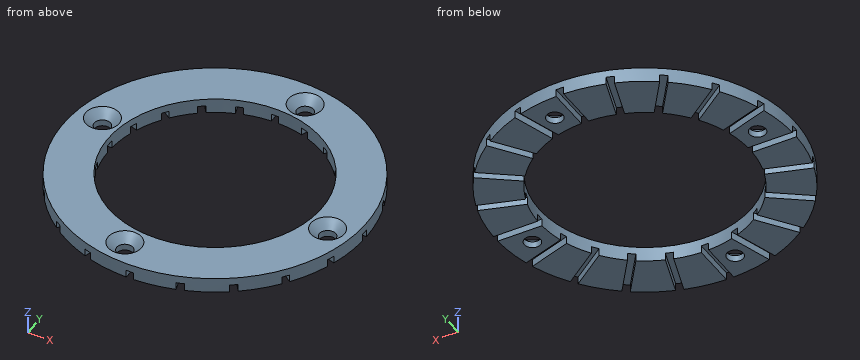
from build123d import *

# Parameters (mm, degrees)
F0_R           = 101.374
F0_R_2         = 71.394
F1_DEPTH       = 10
F3_DEPTH       = 5
F5_D           = 11
F5_CSINK_D     = 22.4
F5_CSINK_ANGLE = 90


with BuildPart() as f1:
    # F0 (on Top) → F1 (new body)
    with BuildSketch(Plane.XY):
        Circle(F0_R)
        Circle(F0_R_2, mode=Mode.SUBTRACT)
    extrude(amount=F1_DEPTH)

    # F2 (on face) → F3 (cut)
    with BuildSketch(Plane(origin=(0, 0, 0), x_dir=(1, 0, 0), z_dir=(0, 0, -1))):
        with BuildLine():
            ThreePointArc((2.5, 101.343168867), (1.2500950523, 101.3662919237), (0, 101.374))
            ThreePointArc((0, 101.374), (-1.2500950523, 101.3662919237), (-2.5, 101.343168867))
            Line((-2.5, 101.343168867), (-2.5, 71.3502153886))
            ThreePointArc((-2.5, 71.3502153886), (0, 71.394), (2.5, 71.3502153886))
            Line((2.5, 71.3502153886), (2.5, 101.343168867))
        make_face()
        with BuildLine():
            ThreePointArc((31.3262879268, 96.4124035626), (30.1349953836, 96.791373217), (28.939120153, 97.1556236189))
            Line((28.939120153, 97.1556236189), (19.6707878167, 68.6306297703))
            ThreePointArc((19.6707878167, 68.6306297703), (22.0619592964, 67.8997289244), (24.4260703981, 67.0855447985))
            Line((24.4260703981, 67.0855447985), (33.6944027344, 95.610538647))
            ThreePointArc((33.6944027344, 95.610538647), (32.5128174779, 96.0187719961), (31.3262879268, 96.4124035626))
        make_face()
        with BuildLine():
            Line((57.5454775947, 83.4578090079), (39.9160618674, 59.1929999324))
            ThreePointArc((39.9160618674, 59.1929999324), (41.9643403022, 57.7589592964), (43.9611468392, 56.254073671))
            Line((43.9611468392, 56.254073671), (61.5905625665, 80.5188827465))
            ThreePointArc((61.5905625665, 80.5188827465), (60.592959405, 81.2722655433), (59.5861417437, 82.0132890945))
            ThreePointArc((59.5861417437, 82.0132890945), (58.5702631175, 82.7418404095), (57.5454775947, 83.4578090079))
        make_face()
        with BuildLine():
            Line((80.5188827465, 61.5905625665), (56.254073671, 43.9611468392))
            ThreePointArc((56.254073671, 43.9611468392), (57.7589592964, 41.9643403022), (59.1929999324, 39.9160618674))
            Line((59.1929999324, 39.9160618674), (83.4578090079, 57.5454775947))
            ThreePointArc((83.4578090079, 57.5454775947), (82.7418395043, 58.5702643962), (82.0132872528, 59.5861442786))
            ThreePointArc((82.0132872528, 59.5861442786), (81.2722646069, 60.592960661), (80.5188827465, 61.5905625665))
        make_face()
        with BuildLine():
            Line((95.610538647, 33.6944027344), (67.0855447985, 24.4260703981))
            ThreePointArc((67.0855447985, 24.4260703981), (67.8997289244, 22.0619592964), (68.6306297703, 19.6707878167))
            Line((68.6306297703, 19.6707878167), (97.1556236189, 28.939120153))
            ThreePointArc((97.1556236189, 28.939120153), (96.7913734751, 30.1349945547), (96.4124040992, 31.3262862756))
            ThreePointArc((96.4124040992, 31.3262862756), (96.0187722746, 32.5128166557), (95.610538647, 33.6944027344))
        make_face()
        with BuildLine():
            Line((101.343168867, 2.5), (71.3502153886, 2.5))
            ThreePointArc((71.3502153886, 2.5), (71.3830530079, 1.2501916945), (71.394, 0))
            ThreePointArc((71.394, 0), (71.3830530079, -1.2501916945), (71.3502153886, -2.5))
            Line((71.3502153886, -2.5), (101.343168867, -2.5))
            ThreePointArc((101.343168867, -2.5), (101.3662919237, -1.2500950523), (101.374, 0))
            ThreePointArc((101.374, 0), (101.3662919237, 1.2500950523), (101.343168867, 2.5))
        make_face()
        with BuildLine():
            Line((97.1556236189, -28.939120153), (68.6306297703, -19.6707878167))
            ThreePointArc((68.6306297703, -19.6707878167), (67.8997289244, -22.0619592964), (67.0855447985, -24.4260703981))
            Line((67.0855447985, -24.4260703981), (95.610538647, -33.6944027344))
            ThreePointArc((95.610538647, -33.6944027344), (96.0187719961, -32.5128174779), (96.4124035626, -31.3262879268))
            ThreePointArc((96.4124035626, -31.3262879268), (96.791373217, -30.1349953836), (97.1556236189, -28.939120153))
        make_face()
        with BuildLine():
            Line((83.4578090079, -57.5454775947), (59.1929999324, -39.9160618674))
            ThreePointArc((59.1929999324, -39.9160618674), (57.7589592964, -41.9643403022), (56.254073671, -43.9611468392))
            Line((56.254073671, -43.9611468392), (80.5188827465, -61.5905625665))
            ThreePointArc((80.5188827465, -61.5905625665), (81.2722651856, -60.5929598848), (82.013288391, -59.586142712))
            ThreePointArc((82.013288391, -59.586142712), (82.7418400637, -58.5702636059), (83.4578090079, -57.5454775947))
        make_face()
        with BuildLine():
            Line((61.5905625665, -80.5188827465), (43.9611468392, -56.254073671))
            ThreePointArc((43.9611468392, -56.254073671), (41.9643403022, -57.7589592964), (39.9160618674, -59.1929999324))
            Line((39.9160618674, -59.1929999324), (57.5454775947, -83.4578090079))
            ThreePointArc((57.5454775947, -83.4578090079), (58.5702643962, -82.7418395043), (59.5861442786, -82.0132872528))
            ThreePointArc((59.5861442786, -82.0132872528), (60.592960661, -81.2722646069), (61.5905625665, -80.5188827465))
        make_face()
        with BuildLine():
            Line((33.6944027344, -95.610538647), (24.4260703981, -67.0855447985))
            ThreePointArc((24.4260703981, -67.0855447985), (22.0619592964, -67.8997289244), (19.6707878167, -68.6306297703))
            Line((19.6707878167, -68.6306297703), (28.939120153, -97.1556236189))
            ThreePointArc((28.939120153, -97.1556236189), (30.1349953836, -96.791373217), (31.3262879268, -96.4124035626))
            ThreePointArc((31.3262879268, -96.4124035626), (32.5128174779, -96.0187719961), (33.6944027344, -95.610538647))
        make_face()
        with BuildLine():
            ThreePointArc((2.5, -71.3502153886), (0, -71.394), (-2.5, -71.3502153886))
            Line((-2.5, -71.3502153886), (-2.5, -101.343168867))
            ThreePointArc((-2.5, -101.343168867), (-1.2500950523, -101.3662919237), (0, -101.374))
            ThreePointArc((0, -101.374), (1.2500950523, -101.3662919237), (2.5, -101.343168867))
            Line((2.5, -101.343168867), (2.5, -71.3502153886))
        make_face()
        with BuildLine():
            ThreePointArc((-19.6707878167, -68.6306297703), (-22.0619592964, -67.8997289244), (-24.4260703981, -67.0855447985))
            Line((-24.4260703981, -67.0855447985), (-33.6944027344, -95.610538647))
            ThreePointArc((-33.6944027344, -95.610538647), (-32.5128191824, -96.018771419), (-31.3262913498, -96.4124024505))
            ThreePointArc((-31.3262913498, -96.4124024505), (-30.1349971018, -96.791372682), (-28.939120153, -97.1556236189))
            Line((-28.939120153, -97.1556236189), (-19.6707878167, -68.6306297703))
        make_face()
        with BuildLine():
            ThreePointArc((-39.9160618674, -59.1929999324), (-41.9643403022, -57.7589592964), (-43.9611468392, -56.254073671))
            Line((-43.9611468392, -56.254073671), (-61.5905625665, -80.5188827465))
            ThreePointArc((-61.5905625665, -80.5188827465), (-60.5929601813, -81.2722649646), (-59.5861433104, -82.0132879563))
            ThreePointArc((-59.5861433104, -82.0132879563), (-58.5702639078, -82.7418398501), (-57.5454775947, -83.4578090079))
            Line((-57.5454775947, -83.4578090079), (-39.9160618674, -59.1929999324))
        make_face()
        with BuildLine():
            ThreePointArc((-56.254073671, -43.9611468392), (-57.7589592964, -41.9643403022), (-59.1929999324, -39.9160618674))
            Line((-59.1929999324, -39.9160618674), (-83.4578090079, -57.5454775947))
            ThreePointArc((-83.4578090079, -57.5454775947), (-82.7418404095, -58.5702631175), (-82.0132890945, -59.5861417437))
            ThreePointArc((-82.0132890945, -59.5861417437), (-81.2722655433, -60.592959405), (-80.5188827465, -61.5905625665))
            Line((-80.5188827465, -61.5905625665), (-56.254073671, -43.9611468392))
        make_face()
        with BuildLine():
            ThreePointArc((-67.0855447985, -24.4260703981), (-67.8997289244, -22.0619592964), (-68.6306297703, -19.6707878167))
            Line((-68.6306297703, -19.6707878167), (-97.1556236189, -28.939120153))
            ThreePointArc((-97.1556236189, -28.939120153), (-96.791373217, -30.1349953836), (-96.4124035626, -31.3262879268))
            ThreePointArc((-96.4124035626, -31.3262879268), (-96.0187719961, -32.5128174779), (-95.610538647, -33.6944027344))
            Line((-95.610538647, -33.6944027344), (-67.0855447985, -24.4260703981))
        make_face()
        with BuildLine():
            ThreePointArc((-71.3502153886, -2.5), (-71.394, 0), (-71.3502153886, 2.5))
            Line((-71.3502153886, 2.5), (-101.343168867, 2.5))
            ThreePointArc((-101.343168867, 2.5), (-101.3662919237, 1.2500950523), (-101.374, 0))
            ThreePointArc((-101.374, 0), (-101.3662919237, -1.2500950523), (-101.343168867, -2.5))
            Line((-101.343168867, -2.5), (-71.3502153886, -2.5))
        make_face()
        with BuildLine():
            ThreePointArc((-68.6306297703, 19.6707878167), (-67.8997289244, 22.0619592964), (-67.0855447985, 24.4260703981))
            Line((-67.0855447985, 24.4260703981), (-95.610538647, 33.6944027344))
            ThreePointArc((-95.610538647, 33.6944027344), (-96.0187717709, 32.5128181431), (-96.4124031286, 31.3262892627))
            ThreePointArc((-96.4124031286, 31.3262892627), (-96.7913730082, 30.1349960542), (-97.1556236189, 28.939120153))
            Line((-97.1556236189, 28.939120153), (-68.6306297703, 19.6707878167))
        make_face()
        with BuildLine():
            ThreePointArc((-59.1929999324, 39.9160618674), (-57.7589592964, 41.9643403022), (-56.254073671, 43.9611468392))
            Line((-56.254073671, 43.9611468392), (-80.5188827465, 61.5905625665))
            ThreePointArc((-80.5188827465, 61.5905625665), (-81.272264828, 60.5929603645), (-82.0132876875, 59.5861436802))
            ThreePointArc((-82.0132876875, 59.5861436802), (-82.741839718, 58.5702640943), (-83.4578090079, 57.5454775947))
            Line((-83.4578090079, 57.5454775947), (-59.1929999324, 39.9160618674))
        make_face()
        with BuildLine():
            ThreePointArc((-43.9611468392, 56.254073671), (-41.9643403022, 57.7589592964), (-39.9160618674, 59.1929999324))
            Line((-39.9160618674, 59.1929999324), (-57.5454775947, 83.4578090079))
            ThreePointArc((-57.5454775947, 83.4578090079), (-58.5702643962, 82.7418395043), (-59.5861442786, 82.0132872528))
            ThreePointArc((-59.5861442786, 82.0132872528), (-60.592960661, 81.2722646069), (-61.5905625665, 80.5188827465))
            Line((-61.5905625665, 80.5188827465), (-43.9611468392, 56.254073671))
        make_face()
        with BuildLine():
            Line((-19.6707878167, 68.6306297703), (-28.939120153, 97.1556236189))
            ThreePointArc((-28.939120153, 97.1556236189), (-30.134995798, 96.791373088), (-31.3262887525, 96.4124032944))
            ThreePointArc((-31.3262887525, 96.4124032944), (-32.5128178891, 96.0187718569), (-33.6944027344, 95.610538647))
            Line((-33.6944027344, 95.610538647), (-24.4260703981, 67.0855447985))
            ThreePointArc((-24.4260703981, 67.0855447985), (-22.0619592964, 67.8997289244), (-19.6707878167, 68.6306297703))
        make_face()
    extrude(amount=-F3_DEPTH, mode=Mode.SUBTRACT)

    # F5 (through all)
    with Locations(Plane.XY.offset(10)):
        with Locations((13.2969295284, 83.9535089506), (83.9535089506, -13.2969295284), (-83.9535089506, 13.2969295284), (-13.2969295284, -83.9535089506)):
            CounterSinkHole(F5_D / 2, F5_CSINK_D / 2, counter_sink_angle=F5_CSINK_ANGLE)


solid = f1.part
Here's how the part is built. I have some questions about the finished solid (model axes, mm). Round coordinates to 2 decimals unless told otherwise and drop trailing zeros. Loops run counter-clockwise (first coordinate to the right, second up) from the corner with the lowest first, then second, coordinate; pieces in that order, holes last. Notation, with made-up numbers: (-38, 35.25) - (8, 35.25) arc R17 cw to (8, 64.25) - close; hole circle Ø9 at (47, 69.25). An arc over 180 degrees is marked (long way). One line per question, with ' | ' between items. Start each with the question number.
Q1. Please list where these lines run through material, in increasing order: line 1 (Y direction, x = 83.5, z = 4.75); line 2 (X direction, y = -82.5, z = 3.5); line 3 (X direction, y = 87, z = 1). Write a range as [from, to].
Q2. I want a section at A-A (y = -52). Write out the boundary of the cut face in (x, z), then the cut area to 3 significant figures.
Q3. I want a section at B-B (z = 7.25). Write out the boundary of the cut face in (x, y), then the cut area to 3 significant figures.
Q4. I want a section at C-C (x = 64.5). Write out the boundary of the cut face in (y, z), then the cut area to 3 significant figures.
Q5. Will these pins go through, and if not, where does the flat tip stop? pin 1 (2.5 mm diameter, centred on y = 91, z = 3.5, fed in from -X); pin 2 (4 mm diameter, centred on x = -65.5, z = 8.5, fed in from +Y); pin 3 (2 mm diameter, centred on y = -61.5, z = 1.5, fed in from -X).
Response values:
1) line 1: y = [-57.48, -29.76], [-24.5, -19.23], [-7.36, -2.5], [2.5, 24.5], [29.76, 57.48] | line 2: x = [-56.85, -29.43], [-24.18, -18.6], [-7.99, -2.5], [2.5, 24.18], [29.43, 56.85] | line 3: x = [-52.04, -30.9], [-25.64, -2.5], [2.5, 8.72], [17.88, 25.64], [30.9, 52.04]
2) outline: (-87.02, 0) - (-75.83, 0) - (-75.83, 5) - (-67.32, 5) - (-67.32, 0) - (-48.92, 0) - (-48.92, 10) - (-87.02, 10) - close; (48.92, 0) - (67.32, 0) - (67.32, 5) - (75.83, 5) - (75.83, 0) - (87.02, 0) - (87.02, 10) - (48.92, 10) - close | area: 677 mm²
3) outline: circle Ø202.75 at (0, 0); hole circle Ø16.9 at (-83.95, 13.3); hole circle Ø142.79 at (0, 0); hole circle Ø16.9 at (-13.3, -83.95); hole circle Ø16.9 at (13.3, 83.95); hole circle Ø16.9 at (83.95, -13.3) | area: 15,400 mm²
4) outline: (-78.21, 0) - (-49.95, 0) - (-49.95, 5) - (-43.77, 5) - (-43.77, 0) - (-30.61, 0) - (-30.61, 10) - (-78.21, 10) - close; (30.61, 0) - (43.77, 0) - (43.77, 5) - (49.95, 5) - (49.95, 0) - (78.21, 0) - (78.21, 10) - (30.61, 10) - close | area: 890 mm²
5) pin 1: stops at x = -47.13 | pin 2: stops at y = 79.02 | pin 3: stops at x = -80.52
